Geometry check sheet. Reference: the model listing, model coordinates, mm. Round coordinates to 2 decimals unless told otherwise and drop trailing zeros. Write each loop counter-clockwise with the first axis right and the second up, starting at its lowest first coordinate (ties: lowest second). Pieces come first, ordered by that corner, then holes.
from build123d import *

# Parameters (mm, degrees)
SWEEP1_PROFILE_R                           = 8
HOLLOW_TUBE_OD_AND_WALL_PROVISIONAL_PROF_R = 6


with BuildPart() as part:
    # Sweep1: sweep along a curve in space
    with BuildLine() as sweep1_path:
        Line((0, 0, 0), (0, 152.000001606, 0))
        ThreePointArc((0, 152.000001606, 0), (0, 169.677670568, -7.322330568), (0, 177, -25))
        Line((0, 177, -25), (0, 177, -141))
    # Sweep1 profile (on start of the path) → Sweep1 (sweep)
    with BuildSketch(Plane.ZX):
        Circle(SWEEP1_PROFILE_R)
    sweep(path=sweep1_path.line)

    # Hollow_tube_OD_and_wall_PROVISIONAL: sweep along a curve in space
    with BuildLine() as hollow_tube_od_and_wall_provisional_path:
        Line((0, 0, 0), (0, 152.000001606, 0))
        ThreePointArc((0, 152.000001606, 0), (0, 169.677670568, -7.322330568), (0, 177, -25))
        Line((0, 177, -25), (0, 177, -141))
    # Hollow_tube_OD_and_wall_PROVISIONAL prof (on start of the path) → Hollow_tube_OD_and_wall_PROVISIONAL (sweep, cut)
    with BuildSketch(Plane.ZX):
        Circle(HOLLOW_TUBE_OD_AND_WALL_PROVISIONAL_PROF_R)
    sweep(path=hollow_tube_od_and_wall_provisional_path.line, mode=Mode.SUBTRACT)


solid = part.part
1. Section check A-A (y = 45.5). Record the cut outline in (x, z).
2. Depth check by flat-ended pin: pin 1 Ø3 at (x, z) = (3.5, -119) entering from +Y; pin 2 Ø1.5 at (x, y) = (3, 72.5) entering from -Z; pin 3 Ø4 at (x, z) = (1, -100.5) entering from -Y. Enter the tip coordinate at first touch or a pass-through.
3. Scan lines: line 1 along X through (y, z) = (59, 0); line 2 along Y through (x, z) = (4.5, -120); line 3 along Y through (x, z) = (-3.25, -123). Record each from-to range of solid material in increasing order.
4. Release check for a two-part mould opening along Z. For faces 1 (the face through (-6, 179, -141)), 2 (the face through (0, 77, -6)), 3 (the face through (-7.81, 77.06, -1.73)) record: +Z half, -Z half, draft (parallel to the pull), parting line (faces both ways), or undercut.
Results below:
1. outline: circle Ø16 at (0, 0); hole circle Ø12 at (0, 0)
2. pin 1: stops at y = 184.75
2. pin 2: stops at z = -7.68
2. pin 3: stops at y = 169
3. line 1: x = -8 to -6, 6 to 8
3. line 2: y = 170.39 to 173.03, 180.97 to 183.61
3. line 3: y = 169.69 to 171.96, 182.04 to 184.31
4. face 1: -Z half
4. face 2: undercut
4. face 3: parting line
